Could you check a few things on this model? Use its own coordinates, in mm. A direction names the side the tool comes from. Round coordinates to 2 decimals unless told otherwise and drop trailing zeros. Loops run counter-clockwise (first coordinate to the right, second up) from the corner with the lowest first, then second, coordinate; pieces in that order, holes last.
Autodesk Inventor part; units mm, degrees
ref_plane "Work Plane1" through (18, 0, 0) normal (1, 0, 0) x (0, 0, -1)
ref_plane "Work Plane2" through (21, 7.7, 7.5) normal (1, 0, 0) x (0, 0, -1)
ref_plane "YZ Plane" through (0, 0, 0) normal (1, 0, 0) x (0, 1, 0)
sketch "Sketch1" plane through (0, 0, 0) normal (0, 0, 1) x (1, 0, 0)
  line L0 (0, 0) -> (0, 2.5)
  line L1 (0, 2.5) -> (8.5, 2.5)
  line L2 (8.5, 2.5) -> (8.5, 12.7)
  line L3 (8.5, 12.7) -> (0, 12.7)
  line L4 (0, 12.7) -> (0, 15.2)
  line L5 (0, 15.2) -> (15, 15.2)
  line L6 (15, 15.2) -> (15, 0)
  line L7 (15, 0) -> (0, 0)
  dimension "d0" = 2.5
  dimension "d1" = 8.5
  dimension "d2" = 10.2
  dimension "d3" = 2.5
  dimension "d4" = 15
extrude "Extrusion1" add sketch "Sketch1" along normal blind 15
ref_plane "Work Plane1" through (18, 0, 0) normal (1, 0, 0) x (0, 0, -1)
sketch "Sketch3" plane through (15, 0, 0) normal (1, 0, 0) x (0, 0, -1)
  line L0 (0, 15.2) -> (-15, 15.2)
  line L1 (-15, 15.2) -> (0, 15.2)
  line L2 (0, 0) -> (-15, 0)
  line L3 (0, 15.2) -> (0, 0)
  line L4 (-15, 2.5) -> (-15, 0)
  line L5 (0, 0) -> (-15, 0)
  line L6 (-15, 15.2) -> (-15, 12.7)
  line L7 (-15, 0) -> (-15, 15.2)
sketch "Sketch4" plane through (18, 0, 0) normal (1, 0, 0) x (0, 0, -1)
  circle A0 centre (-7.5, 7.7) radius 9
  line L0 (0, 15.2) -> (-15, 15.2)
  line L1 (-15, 0) -> (-15, 15.2)
  point P0 (0, 0)
  dimension "d10" = 18
  dimension "d11" = 7.5
  dimension "d12" = 7.5
ref_plane "Work Plane2" through (21, 7.7, 7.5) normal (1, 0, 0) x (0, 0, -1)
sketch "Sketch5" plane through (21, 7.7, 7.5) normal (1, 0, 0) x (0, 0, -1)
  circle A0 centre (0, 0) radius 12
  point P0 (7.5, -7.7)
  dimension "d18" = 24
sketch "Sketch4 outline for Loft2" plane through (18, 0, 0) normal (1, 0, 0) x (0, 0, -1)
  circle A0 centre (-7.5, 7.7) radius 9
sketch "Sketch5 outline for Loft2" plane through (21, 7.7, 7.5) normal (1, 0, 0) x (0, 0, -1)
  circle A0 centre (0, 0) radius 12
loft "Loft2" add profiles "Sketch4 outline for Loft2", "Sketch5 outline for Loft2" section 1 edges at (15, 7.6, 0) (15, 15.2, 7.5) (15, 7.6, 15) (15, 0, 7.5)
sketch "Sketch6" plane through (21, 7.7, 7.5) normal (1, 0, 0) x (0, 0, -1)
  circle A0 centre (0, 0) radius 7.75
  circle A1 centre (0, 0) radius 12
  point P0 (7.5, -7.7)
  dimension "d25" = 15.5
extrude "Extrusion2" add sketch "Sketch6" along normal blind 28
ref_plane "Work Plane3" through (0, 0, 7.5) normal (0, 0, 1) x (1, 0, 0)
sketch "Sketch7" plane through (0, 0, 7.5) normal (0, 0, 1) x (1, 0, 0)
  line L0 (21, 19.7) -> (49, 19.7)
  line L1 (49, 19.7) -> (21, 19.7)
  line L2 (21, 16.241288) -> (21, -0.841288)
  line L3 (21, 15.217594) -> (49, 15.217594)
  line L4 (49, -4.3) -> (49, 19.7)
  line L5 (49, 15.217594) -> (49, 19.7)
  line L6 (21, 19.7) -> (21, 16.241288)
  line L7 (21, 19.7) -> (21, 15.217594)
  point P0 (0, 0)
extrude "Extrusion3" cut sketch "Sketch7" against normal mid plane 2
sketch "Sketch8" plane through (49, 7.7, 7.5) normal (1, 0, 0) x (0, 0, -1)
  point P0 (7.5, -7.7)
sketch "Sketch10" plane through (49, 7.7, 7.5) normal (1, 0, 0) x (0, 0, -1)
  arc A0 (-1, 11.958261) -> (-8.428903, 8.541288) centre (0, 0) ccw
  line L0 (-1, 11.958261) -> (-1, 20.958261)
  line L1 (-1, 20.958261) -> (-6, 20.958261)
  line L2 (-6, 20.958261) -> (-6, 10.392305)
  arc A1 (8.428903, 8.541288) -> (1, 11.958261) centre (0, 0) ccw
  line L3 (1, 11.958261) -> (1, 20.958261)
  line L4 (1, 20.958261) -> (6, 20.958261)
  line L5 (6, 20.958261) -> (6, 10.392305)
  arc A2 (-1, 11.958261) -> (-6, 10.392305) centre (0, 0) ccw
  line L6 (1, 7.685213) -> (1, 11.958261)
  arc A3 (6, 10.392305) -> (1, 11.958261) centre (0, 0) ccw
  point P0 (7.5, -7.7)
  dimension "d33" = 9
  dimension "d34" = 5
  dimension "d35" = 5
extrude "Extrusion4" add sketch "Sketch10" against normal blind 15
sketch "Sketch11" plane through (49, 18.092305, 1.5) normal (0, 0, -1) x (-1, 0, 0)
  circle A0 centre (7.5, 6.35) radius 1.75
  point P0 (49, -18.092305)
  dimension "d38" = 3.5
extrude "Extrusion5" cut sketch "Sketch11" against normal through all
sketch "Sketch12" plane through (49, 18.092305, 1.5) normal (0, 0, -1) x (-1, 0, 0)
  circle A0 centre (7.5, 6.35) radius 1.75
  circle A1 centre (7.5, 6.35) radius 3
  point P0 (49, -18.092305)
  dimension "d41" = 6
extrude "Extrusion6" cut sketch "Sketch12" against normal blind 2.5 contours A0 | A1
sketch "Sketch13" plane through (0, 0, 8.5) normal (0, 0, -1) x (-1, 0, 0)
  point P0 (0, 0)
sketch "Sketch14" plane through (49, 18.092305, 13.5) normal (0, 0, 1) x (1, 0, 0)
  circle A0 centre (-7.5, 6.35) radius 1.75
  line L0 (-3.920428, 6.35) -> (-5.710214, 3.25)
  line L1 (-5.710214, 3.25) -> (-9.289786, 3.25)
  line L2 (-9.289786, 3.25) -> (-11.079572, 6.35)
  line L3 (-11.079572, 6.35) -> (-9.289786, 9.45)
  line L4 (-9.289786, 9.45) -> (-5.710214, 9.45)
  line L5 (-5.710214, 9.45) -> (-3.920428, 6.35)
  point P0 (-49, -18.092305)
  dimension "d44" = 6.2
extrude "Extrusion7" cut sketch "Sketch14" against normal blind 2.5
sketch "Sketch15" plane through (0, 2.5, 0) normal (0, 1, 0) x (1, 0, 0)
  circle A0 centre (4.3, -7.5) radius 2.25
  line L0 (8.5, 0) -> (8.5, -15)
  point P0 (0, 0)
  dimension "d47" = 4.5
  dimension "d48" = 4.2
extrude "Extrusion8" cut sketch "Sketch15" along normal through all both and the other way through all
properties part number "Arm connection"
Item 1: Will these pins go through, and if not, where does the flat tip stop? pin 1 (2.5 mm diameter, centred on x = 6.5, z = 4.5, fed in from -Y); pin 2 (2 mm diameter, centred on x = 19, y = 11, fed in from +Z); pin 3 (12.5 mm diameter, centred on y = 7.5, z = 7, fed in from +X).
Results list:
pin 1: stops at y = 0
pin 2: stops at z = 17.67
pin 3: stops at x = 21
Item 2: If we section it at A-A, the plane x = 4.3: Please give me the cut outline in (y, z).
Results list:
outline: (0, 0) - (2.5, 0) - (2.5, 5.25) - (0, 5.25) - close; (0, 9.75) - (2.5, 9.75) - (2.5, 15) - (0, 15) - close; (12.7, 0) - (15.2, 0) - (15.2, 5.25) - (12.7, 5.25) - close; (12.7, 9.75) - (15.2, 9.75) - (15.2, 15) - (12.7, 15) - close
Item 3: If I drill on line 1 along Z through (x, y) = (4.3, 1.1); line 2 along Y through (x, z) = (42, 10.5); line 3 along X through (y, z) = (1.7, 7.5), over which ranges is the centre line in solid material (lowest first)?
Results list:
line 1: z = 0 to 5.25, 9.75 to 15
line 2: y = -3.92 to 0.55, 14.85 to 22.77, 26.12 to 28.66
line 3: x = 0 to 2.05, 6.55 to 21
Item 4: If we section it at B-B, the plane x = 41.5: Please give me the cut outline in (y, z), then the cut area to 3 significant figures.
Results list:
outline: (15.39, 6.5) arc R7.75 cw (long way) to (15.39, 8.5) - (22.69, 8.5) - (22.69, 11) - (21.34, 11) - (21.34, 13.5) - (18.09, 13.5) arc R12 ccw (long way) to (18.09, 1.5) - (21.44, 1.5) - (21.44, 4) - (22.69, 4) - (22.69, 6.5) - close; (26.19, 4) - (27.44, 4) - (27.44, 1.5) - (28.66, 1.5) - (28.66, 6.5) - (26.19, 6.5) - close; (26.19, 8.5) - (28.66, 8.5) - (28.66, 13.5) - (27.54, 13.5) - (27.54, 11) - (26.19, 11) - close
area: 303 mm2
Item 5: For faces 1 (the flat face through (42, 21, 13.5)), 2 (the flat face through (9, 8, 15)), 3 (the flat face through (44.172, 26.014, 12.268)), 4 (the cylindrical face through (34.804, -0.043, 7.173)), 5 (the flat face through (6.1, 2.5, 9.1)), which set-ups out of +Z, -Z, +X, -X, +Y, -Y let a thin tool reach every point of the face, with its end or its side?
Results list:
face 1: +Z, +X, -X, +Y
face 2: +Z, -X, +Y, -Y
face 3: +Z
face 4: +X
face 5: +Z, -Z, -X
Item 6: If we section it at C-C, the plane z = 7.5: Count the separate pieces of the cut face and the enclosed holes in it, then the cut area to 3 significant figures.
Results list:
separate pieces: 3
enclosed holes: 0
area: 349 mm2
Item 7: We'd pull the mould along Y, two halves only. Please class faces 6 (the flat face through (34, 23, 11)), 7 (the flat face through (2, 12.7, 9)): released by +Y, released by -Y, zero draft, split by the parting line, or undercut.
Results list:
face 6: zero draft
face 7: undercut
Item 8: If we section it at D-D, the plane x = 35.5: Please give me the cut outline in (y, z).
Results list:
outline: (15.39, 6.5) arc R7.75 cw (long way) to (15.39, 8.5) - (28.66, 8.5) - (28.66, 13.5) - (18.09, 13.5) arc R12 ccw (long way) to (18.09, 1.5) - (28.66, 1.5) - (28.66, 6.5) - close
